Part print with two shaded views. Sizes in mm from the minimum x, y, z corner. A direction names the side the tool comes from. Round coordinates to 2 decimals unless told otherwise and drop trailing zeros. Loops run counter-clockwise (first coordinate to the right, second up) from the corner with the lowest first, then second, coordinate; pieces in that order, holes last.
(1) Probe probe 1 along Y at (x, z) = (10, 1.45); probe 2 along X at (y, z) = (7.25, 1.8); probe 3 along Y at (x, z) = (9.5, 0.8). List the from-to ranges inside material, lowest first.
(2) Cut at C-C on y = 10. List the corners of the cut face in (x, z), then the cut area to 3 significant figures.
(3) Cut at B-B on x = 16. List the corners of the cut face in (y, z), then the cut area to 3 significant figures.
(4) Cut at D-D on z = 2.25. List the corners of the cut face in (x, y).
(5) Mould opens along X. For the marked faces 3, 4, 5 and 6 say: +X half, -X half, draft (parallel to the pull), parting line (faces both ways), or undercut.
(6) Tool access for the marked faces 1 and 2: list every direction of +Z, -Z, +X, -X, +Y, -Y with a clear straight run to the whole face (end or side of a thin tool).
(7) Flat gauge pin, fed straight in: pin 1 (4 mm diameter, centred on x = 5, y = 16, fed in from -Z). Where does the tip first touch, or does it go through?
(8) Cut at A-A on x = 10. List the corners of the cut face in (y, z), then the cut area to 3 significant figures.
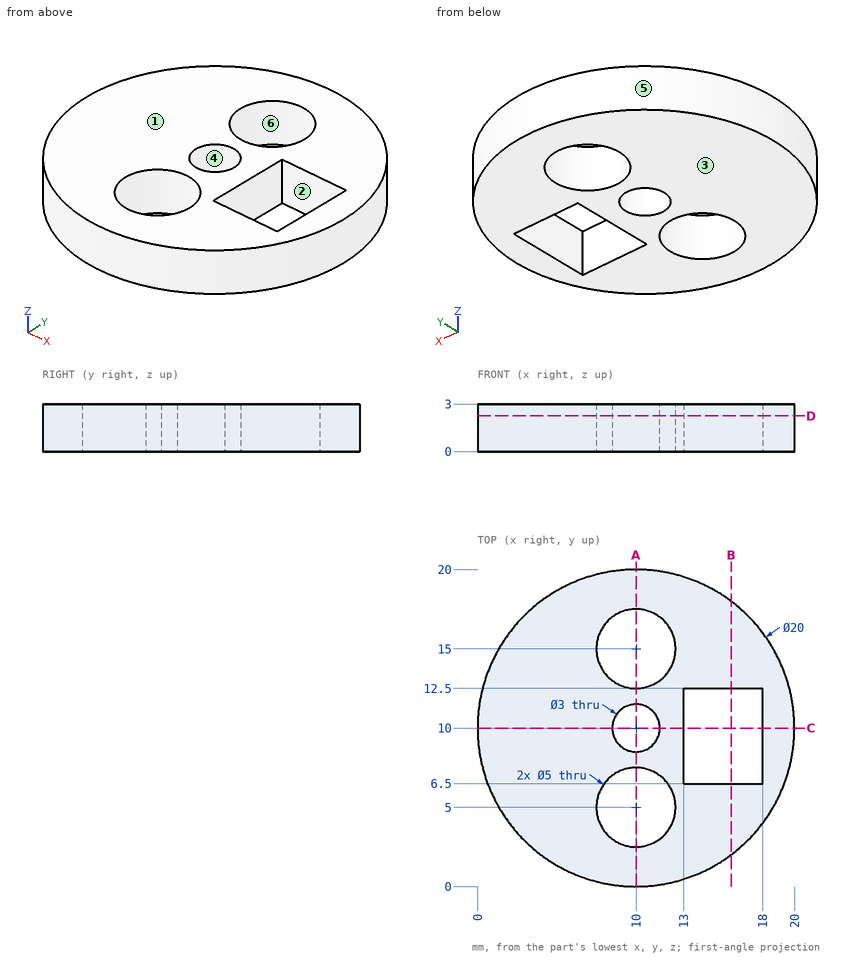
Final values:
1. probe 1: y = 0 to 2.5, 7.5 to 8.5, 11.5 to 12.5, 17.5 to 20
1. probe 2: x = 0.39 to 8.91, 11.09 to 13, 18 to 19.61
1. probe 3: y = 0.01 to 2.55, 7.45 to 8.59, 11.41 to 12.55, 17.45 to 19.99
2. outline: (0, 0) - (8.5, 0) - (8.5, 3) - (0, 3) - close; (11.5, 0) - (13, 0) - (13, 3) - (11.5, 3) - close; (18, 0) - (20, 0) - (20, 3) - (18, 3) - close
2. area: 36.0 mm2
3. outline: (2, 0) - (6.5, 0) - (6.5, 3) - (2, 3) - close; (12.5, 0) - (18, 0) - (18, 3) - (12.5, 3) - close
3. area: 30.0 mm2
4. outline: circle Ø20 at (10, 10); hole circle Ø5 at (10, 5); hole circle Ø5 at (10, 15); hole circle Ø3 at (10, 10); hole (13, 6.5) - (18, 6.5) - (18, 12.5) - (13, 12.5) - close
5. face 3: draft
5. face 4: undercut
5. face 5: parting line
5. face 6: undercut
6. face 1: +Z, +X, -X, +Y, -Y
6. face 2: +Z, -Z
7. pin 1: stops at z = 0
8. outline: (0, 0) - (2.5, 0) - (2.5, 3) - (0, 3) - close; (7.5, 0) - (8.5, 0) - (8.5, 3) - (7.5, 3) - close; (11.5, 0) - (12.5, 0) - (12.5, 3) - (11.5, 3) - close; (17.5, 0) - (20, 0) - (20, 3) - (17.5, 3) - close
8. area: 21.0 mm2
